```python
from build123d import *

# Parameters (mm, degrees)
SKETCH1_W                = 34
SKETCH1_H                = 28.5
BOSS_EXTRUDE1_DEPTH      = 22.7
SKETCH3_R                = 12.6
CUT_EXTRUDE1_DEPTH       = 19
SKETCH5_R                = 1.625
SKETCH5_R_2              = 3.75
CUT_EXTRUDE2_DEPTH       = 30.207233693
BOSS_EXTRUDE2_DEPTH      = 4.93
BOSS_EXTRUDE2_DEPTH_BACK = 3.72
SKETCH7_W                = 8.75
SKETCH7_H                = 12.5
SKETCH8_R                = 1.75
CUT_EXTRUDE3_DEPTH       = 42.018037496
SKETCH9_R                = 3.25
CUT_EXTRUDE4_DEPTH       = 3.175
SKETCH14_R               = 1.75
CUT_EXTRUDE8_DEPTH       = 50


with BuildPart() as part:
    # Sketch1 → Boss-Extrude1 (new body)
    with BuildSketch(Plane.XY):
        Rectangle(SKETCH1_W, SKETCH1_H)
    extrude(amount=BOSS_EXTRUDE1_DEPTH)

    # Sketch3 → Cut-Extrude1 (cut)
    with BuildSketch(Plane.XY.offset(22.7)):
        Circle(SKETCH3_R)
    extrude(amount=-CUT_EXTRUDE1_DEPTH, mode=Mode.SUBTRACT)

    # Sketch5 → Cut-Extrude2 (cut, through all)
    with BuildSketch(Plane.XY.offset(3.7)):
        with Locations((6.01040764, 6.01040764)):
            Circle(SKETCH5_R)
        with Locations((-6.01040764, 6.01040764)):
            Circle(SKETCH5_R)
        with Locations((6.01040764, -6.01040764)):
            Circle(SKETCH5_R)
        with Locations((-6.01040764, -6.01040764)):
            Circle(SKETCH5_R)
        Circle(SKETCH5_R_2)
    extrude(amount=-CUT_EXTRUDE2_DEPTH, mode=Mode.SUBTRACT)

    # Sketch7 → Boss-Extrude2 (add, two sides: drawn at the far end of the back side and taken through both)
    with BuildSketch(Plane.XY.offset(22.7).offset(-BOSS_EXTRUDE2_DEPTH_BACK)):
        with Locations((-21.375, -8)):
            Rectangle(SKETCH7_W, SKETCH7_H)
        with Locations((21.375, -8)):
            Rectangle(SKETCH7_W, SKETCH7_H)
    extrude(amount=BOSS_EXTRUDE2_DEPTH + BOSS_EXTRUDE2_DEPTH_BACK)

    # Sketch8 → Cut-Extrude3 (cut, through all)
    with BuildSketch(Plane(origin=(0, -1.75, 0), x_dir=(1, 0, 0), z_dir=(0, 1, 0))):
        with Locations(Location((21.375, -23.305, 0), (0, 0, 180))):
            Circle(SKETCH8_R)
        with Locations(Location((-21.375, -23.305, 0), (0, 0, 180))):
            Circle(SKETCH8_R)
    extrude(amount=-CUT_EXTRUDE3_DEPTH, mode=Mode.SUBTRACT)

    # Sketch9 → Cut-Extrude4 (cut)
    with BuildSketch(Plane.XZ.offset(14.25)):
        with Locations((-21.375, 23.305)):
            Circle(SKETCH9_R)
        with Locations((21.375, 23.305)):
            Circle(SKETCH9_R)
    extrude(amount=-CUT_EXTRUDE4_DEPTH, mode=Mode.SUBTRACT)

    # Cut-Extrude5 cone 1 section (through the dimple's axis) → Cut-Extrude5 (revolve, cut)
    with BuildSketch(Plane(origin=(-6.01040764, 6.01040764, 0), x_dir=(0, 1, 0), z_dir=(1, 0, 0))):
        Polygon((0, 0), (2.8, 0), (0, 2.8), align=None)
    revolve(axis=Axis((-6.01040764, 6.01040764, 0), (0, 0, 1)), mode=Mode.SUBTRACT)

    # Cut-Extrude5 cone 2 section (through the dimple's axis) → Cut-Extrude5 cone 2 (revolve, cut)
    with BuildSketch(Plane(origin=(-6.01040764, -6.01040764, 0), x_dir=(0, 1, 0), z_dir=(1, 0, 0))):
        Polygon((0, 0), (2.8, 0), (0, 2.8), align=None)
    revolve(axis=Axis((-6.01040764, -6.01040764, 0), (0, 0, 1)), mode=Mode.SUBTRACT)

    # Cut-Extrude5 cone 3 section (through the dimple's axis) → Cut-Extrude5 cone 3 (revolve, cut)
    with BuildSketch(Plane(origin=(6.01040764, -6.01040764, 0), x_dir=(0, 1, 0), z_dir=(1, 0, 0))):
        Polygon((0, 0), (2.8, 0), (0, 2.8), align=None)
    revolve(axis=Axis((6.01040764, -6.01040764, 0), (0, 0, 1)), mode=Mode.SUBTRACT)

    # Cut-Extrude5 cone 4 section (through the dimple's axis) → Cut-Extrude5 cone 4 (revolve, cut)
    with BuildSketch(Plane(origin=(6.01040764, 6.01040764, 0), x_dir=(0, 1, 0), z_dir=(1, 0, 0))):
        Polygon((0, 0), (2.8, 0), (0, 2.8), align=None)
    revolve(axis=Axis((6.01040764, 6.01040764, 0), (0, 0, 1)), mode=Mode.SUBTRACT)

    # Sketch14 → Cut-Extrude8 (cut)
    with BuildSketch(Plane(origin=(132.323959999, 1.25, 25.756345109), x_dir=(1, 0, 0), z_dir=(0, 1, 0))):
        with Locations((-110.733959999, 2.481345109)):
            Circle(SKETCH14_R)
        with Locations((-153.913959999, 2.481345109)):
            Circle(SKETCH14_R)
    extrude(amount=-CUT_EXTRUDE8_DEPTH, mode=Mode.SUBTRACT)


solid = part.part
```
Verification items for the finished model (mm, model axes). A direction names the side the tool comes from. Round coordinates to 2 decimals unless told otherwise and drop trailing zeros. Write each loop counter-clockwise with the first axis right and the second up, starting at its lowest first coordinate (ties: lowest second). Pieces come first, ordered by that corner, then holes.
1. Gauge pin test, flat ends, axial feed: P1, Ø8.5, axis at x = -2, y = 1, coming from the +Z side; P2, Ø6, axis at x = 21.375, z = 23.305, coming from the +Y side; P3, Ø7, axis at x = 21.5, y = -7.5, coming from the -Z side. Record the tip position at first contact, or that the pin passes through.
2. Section check B-B on x = 0. Enter the section's corners in (y, z), plus the area to 3 significant figures.
3. Section check A-A on y = 0. Enter the section's corners in (x, z), plus the area to 3 significant figures.
4. Section check C-C on z = 2.75. Enter the section's corners in (x, y) (3 decimals).
5. Scan lines: L1, parallel to Y at x = -9, z = 19; L2, parallel to X at y = 0.5, z = 17.25; L3, parallel to X at y = 9, z = 19.5. Record each from-to range of solid material in increasing order.
6. Access from +Z, -Z, +X, -X, +Y, -Y to the whole of each face (thin tool, end or side, straight path). Record for faces 4 (the flat face through (-17, -8, 25)), 5 (the cylindrical face through (-19.65, -6.35, 23.59)), 6 (the cylindrical face through (-6.363, -7.597, 2.455)), 7 (the flat face through (25.75, -8, 23)), 8 (the flat face through (-3, -3, 3.7)).
7. Draft check along Y on faces 1 (the cylindrical face through (-22.08, -12.685, 20.132)), 2 (the flat face through (0, 14.25, 11)), 3 (the cylindrical face through (7.56, 6.5, 2.46)). Enter one of: +Y half, -Y half, draft (parallel to the pull), parting line (faces both ways), or undercut.
8. Section check D-D on z = 12.75. Enter the section's corners in (x, y), plus the area to 3 significant figures.
Answer:
1. P1: stops at z = 3.7
1. P2: stops at y = -1.75
1. P3: stops at z = 18.98
2. outline: (-14.25, 0) - (-3.75, 0) - (-3.75, 3.7) - (-12.6, 3.7) - (-12.6, 22.7) - (-14.25, 22.7) - close; (3.75, 0) - (14.25, 0) - (14.25, 22.7) - (12.6, 22.7) - (12.6, 3.7) - (3.75, 3.7) - close
2. area: 140 mm2
3. outline: (-17, 0) - (-3.75, 0) - (-3.75, 3.7) - (-12.6, 3.7) - (-12.6, 22.7) - (-17, 22.7) - close; (3.75, 0) - (17, 0) - (17, 22.7) - (12.6, 22.7) - (12.6, 3.7) - (3.75, 3.7) - close
3. area: 265 mm2
4. outline: (-17, -14.25) - (17, -14.25) - (17, 14.25) - (-17, 14.25) - close; hole circle Ø3.25 at (-6.01, -6.01); hole circle Ø3.25 at (-6.01, 6.01); hole circle Ø7.5 at (0, 0); hole circle Ø3.25 at (6.01, -6.01); hole circle Ø3.25 at (6.01, 6.01)
5. L1: y = -14.25 to -8.82, 8.82 to 14.25
5. L2: x = -17 to -12.59, 12.59 to 17
5. L3: x = -17 to -8.82, 8.82 to 17
6. face 4: +Z, +Y, -Y
6. face 5: +Y, -Y
6. face 6: +Z, -Z
6. face 7: +Z, -Z, +X, +Y, -Y
6. face 8: +Z
7. face 1: draft
7. face 2: +Y half
7. face 3: undercut
8. outline: (-17, -14.25) - (17, -14.25) - (17, 14.25) - (-17, 14.25) - close; hole circle Ø25.2 at (0, 0)
8. area: 470 mm2
